```python
from build123d import *

# Parameters (mm, degrees)
SKETCH1_R                         = 26.4
BOSS_EXTRUDE1_DEPTH               = 0.5
F_4_0_4_DIAMETER_HOLE1_AT_2_COUNT = 2
F_4_0_4_DIAMETER_HOLE1_AT_2_PITCH = 18.85
F_4_0_4_DIAMETER_HOLE1_AT_3_COUNT = 2
F_4_0_4_DIAMETER_HOLE1_AT_3_PITCH = 18.85
F_4_0_4_DIAMETER_HOLE1_AT_4_COUNT = 2
F_4_0_4_DIAMETER_HOLE1_AT_4_PITCH = 18.85
F_4_0_4_DIAMETER_HOLE1_AT_5_COUNT = 2
F_4_0_4_DIAMETER_HOLE1_AT_5_PITCH = 18.85
CHAMFER1_SIZE                     = 0.1
CHAMFER1_SIZE2                    = 0.274747742
SKETCH5_R                         = 5
CUT_EXTRUDE1_DEPTH                = 38.33858594


with BuildPart() as part:
    # Sketch1 → Boss-Extrude1 (new body)
    with BuildSketch(Plane(origin=(0, 0, 0), x_dir=(1, 0, 0), z_dir=(0, 1, 0))):
        with Locations(Location((0, 0, 0), (0, 0, 270))):
            Circle(SKETCH1_R)
    extrude(amount=BOSS_EXTRUDE1_DEPTH)

    # Sketch4 → Ø4.0 (4) Diameter Hole1 (revolve, cut)
    with BuildSketch(Plane(origin=(0, 0.5, 0), x_dir=(0, 0, 1), z_dir=(1, 0, 0))):
        Polygon((0, 0), (0, 0.5), (2, 0.5), (2, 0.027282713), (2.025, 0), align=None)
    f_4_0_4_diameter_hole1 = revolve(axis=Axis((0, 6.85, 0), (0, -1, 0)), mode=Mode.SUBTRACT)

    # Ø4.0 (4) Diameter Hole1 at 2: Ø4.0 (4) Diameter Hole1 ×2
    with Locations(*[(-i * F_4_0_4_DIAMETER_HOLE1_AT_2_PITCH, 0, 0) for i in range(1, F_4_0_4_DIAMETER_HOLE1_AT_2_COUNT)]):
        add(f_4_0_4_diameter_hole1, mode=Mode.SUBTRACT)

    # Ø4.0 (4) Diameter Hole1 at 3: Ø4.0 (4) Diameter Hole1 ×2
    with Locations(*[(0, 0, -i * F_4_0_4_DIAMETER_HOLE1_AT_3_PITCH) for i in range(1, F_4_0_4_DIAMETER_HOLE1_AT_3_COUNT)]):
        add(f_4_0_4_diameter_hole1, mode=Mode.SUBTRACT)

    # Ø4.0 (4) Diameter Hole1 at 4: Ø4.0 (4) Diameter Hole1 ×2
    with Locations(*[(i * F_4_0_4_DIAMETER_HOLE1_AT_4_PITCH, 0, 0) for i in range(1, F_4_0_4_DIAMETER_HOLE1_AT_4_COUNT)]):
        add(f_4_0_4_diameter_hole1, mode=Mode.SUBTRACT)

    # Ø4.0 (4) Diameter Hole1 at 5: Ø4.0 (4) Diameter Hole1 ×2
    with Locations(*[(0, 0, i * F_4_0_4_DIAMETER_HOLE1_AT_5_PITCH) for i in range(1, F_4_0_4_DIAMETER_HOLE1_AT_5_COUNT)]):
        add(f_4_0_4_diameter_hole1, mode=Mode.SUBTRACT)

    # Chamfer1
    chamfer1_edges = [part.edges().sort_by_distance(p)[0] for p in [
        (0, 0, -26.4),
    ]]
    chamfer1_side = [part.faces().sort_by_distance(p)[0] for p in [
        (0, 0, -25.653295239),
    ]]
    chamfer(chamfer1_edges, length=CHAMFER1_SIZE, length2=CHAMFER1_SIZE2, reference=chamfer1_side[0])

    # Sketch5 → Cut-Extrude1 (cut, through all)
    with BuildSketch(Plane(origin=(0, 0.5, 0), x_dir=(1, 0, 0), z_dir=(0, 1, 0))):
        with Locations((-15.056400691, 15.207392881)):
            Circle(SKETCH5_R)
        with BuildLine():
            ThreePointArc((-18.57425135, 18.760522029), (-21.042056901, 15.943394914), (-23.086392584, 12.805408134))
            Line((-23.086392584, 12.805408134), (-16.76402379, 10.508028737))
            ThreePointArc((-16.76402379, 10.508028737), (-19.940282895, 14.136087779), (-18.57425135, 18.760522029))
        make_face()
        with BuildLine():
            ThreePointArc((-12.466103662, 23.271361359), (-15.683202086, 21.236694007), (-18.57425135, 18.760522029))
            ThreePointArc((-18.57425135, 18.760522029), (-13.892859594, 20.070125869), (-10.311269735, 16.783378987))
            Line((-10.311269735, 16.783378987), (-12.466103662, 23.271361359))
        make_face()
    extrude(amount=-CUT_EXTRUDE1_DEPTH, mode=Mode.SUBTRACT)


solid = part.part
```
Verification items for the finished model (mm, model axes). A direction names the side the tool comes from. Coordinates: 2 decimals unless noted, no trailing zeros. Loops run counter-clockwise (first coordinate to the right, second up) from the corner with the lowest first, then second, coordinate; pieces in that order, holes last. Notation, with made-up numbers: (-33, 36.5) - (-16, 36.5) arc R9 cw to (-16, 48.5) - close; hole circle Ø8 at (0.5, -5). An arc over 180 degrees is marked (long way). Return JSON: item names as keys, results as strings.
1. Mould release check, pull along Z, two halves, no side actions. Record for faces 1 (the cylindrical face through (-11.627, 0.254, -11.569)), 2 (the flat face through (-19.969, 0.254, -11.673)), 3 (the flat face through (0, 0.5, 5)): +Z half, -Z half, draft (parallel to the pull), parting line (faces both ways), or undercut.
Established:
{"face 1": "undercut", "face 2": "-Z half", "face 3": "draft"}
2. Thickness scan on L1, parallel to X at y = 0.3, z = 0; L2, parallel to X at y = 0.4, z = 18.85. Record the ranges inside material, lowest first.
Established:
{"L1": "x = -26.4 to -20.85, -16.85 to -2, 2 to 16.85, 20.85 to 26.4", "L2": "x = -18.48 to -2, 2 to 18.48"}
3. Section check A-A, the plane z = 0. Record the boundary of the cut face in (x, y) (3 decimals), then the cut area to 3 significant figures.
Established:
{"outline": "(-26.4, 0.275) - (-26.3, 0) - (-20.85, 0) - (-20.85, 0.473) - (-20.875, 0.5) - (-26.4, 0.5) - close; (-16.85, 0) - (-2, 0) - (-2, 0.473) - (-2.025, 0.5) - (-16.825, 0.5) - (-16.85, 0.473) - close; (2, 0) - (16.85, 0) - (16.85, 0.473) - (16.825, 0.5) - (2.025, 0.5) - (2, 0.473) - close; (20.85, 0) - (26.3, 0) - (26.4, 0.275) - (26.4, 0.5) - (20.875, 0.5) - (20.85, 0.473) - close", "area": "20.4 mm2"}
4. Section check B-B, the plane x = 0. Record the boundary of the cut face in (y, z) (3 decimals), then the cut area to 3 significant figures.
Established:
{"outline": "(0, -26.3) - (0.275, -26.4) - (0.5, -26.4) - (0.5, -20.875) - (0.473, -20.85) - (0, -20.85) - close; (0, -16.85) - (0.473, -16.85) - (0.5, -16.825) - (0.5, -2.025) - (0.473, -2) - (0, -2) - close; (0, 2) - (0.473, 2) - (0.5, 2.025) - (0.5, 16.825) - (0.473, 16.85) - (0, 16.85) - close; (0, 20.85) - (0.473, 20.85) - (0.5, 20.875) - (0.5, 26.4) - (0.275, 26.4) - (0, 26.3) - close", "area": "20.4 mm2"}
5. Section check C-C, the plane y = 0.15. Record the boundary of the cut face in (x, z).
Established:
{"outline": "(-23.04, -12.79) - (-16.76, -10.51) arc R5 cw to (-10.31, -16.78) - (-12.45, -23.23) arc R26.35 ccw (long way) to start; hole circle Ø4 at (-18.85, 0); hole circle Ø4 at (0, -18.85); hole circle Ø4 at (0, 0); hole circle Ø4 at (0, 18.85); hole circle Ø4 at (18.85, 0)"}
6. Tool access check on faces 4 (the cylindrical face through (-0.601, 0.24, -16.942)), 5 (the flat face through (-11.374, 0.254, -19.982)). Record the directions out of +Z, -Z, +X, -X, +Y, -Y that give a thin tool (end or side, any length) a straight path to the whole face; none if there is none.
Established:
{"face 4": "+Y, -Y", "face 5": "-X, +Y, -Y"}
7. Go/stop test with a flat-tipped pin: pin 1 (3 mm diameter, centred on x = 5.5, z = 11.5, fed in from -Y). Record where the tip stops, or that it passes through.
Established:
{"pin 1": "stops at y = 0"}
